Can you work these out from the model? Positions are in its coordinate system, mm. Face numbers are marked on the shaded views. A direction names the side the tool comes from. Round coordinates to 2 decimals unless told otherwise and drop trailing zeros. Loops run counter-clockwise (first coordinate to the right, second up) from the corner with the lowest first, then second, coordinate; pieces in that order, holes last.
Autodesk Fusion 360 part; units mm, degrees
sketch "Sketch1" plane through (0, 0, 0) normal (0, 0, 1) x (1, 0, 0)
  circle A0 centre (0, -11.5) radius 2 construction
  circle A1 centre (0, 0) radius 12 construction
  circle A2 centre (0, -11.5) radius 1.5
  circle A3 centre (0, 0) radius 8.5
  line L0 (0, 0) -> (8.6603, -5)
  circle A4 centre (0, 0) radius 11.5
  line L1 (0, 0) -> (-8.6603, -5)
  circle A5 centre (0, 0) radius 10
  dimension "d4" = 1.5
  dimension "d5" = -1.5
  dimension "d6" = 2
  dimension "d7" = 0.5
  dimension "d8" = 20
  dimension "d9" = 3
extrude "Extrude1" add sketch "Sketch1" along normal blind 2 contours A2 A4 | A2 A4 | A2 A4 | A3 L0 L1 A5 | A3 L0 L1 | A3 L0 L1 picked at (-8.9789, -3.0313)
sketch "Sketch2" plane through (0, 0, 2) normal (0, 0, 1) x (-1, 0, 0)
  arc A0 (7.3612, 4.25) -> (-7.3612, 4.25) centre (0, 0) ccw
  line L0 (-7.3612, 4.25) -> (-8.6603, 5)
  arc A1 (8.6603, 5) -> (-8.6603, 5) centre (0, 0) ccw
  line L1 (8.6603, 5) -> (7.3612, 4.25)
  arc A2 (-1.4968, 11.4022) -> (1.4968, 11.4022) centre (0, 0) ccw
  arc A3 (1.4968, 11.4022) -> (-1.4968, 11.4022) centre (0, 11.5) ccw
  circle A4 centre (0, 0) radius 5
  dimension "d12" = 10
extrude "Extrude2" add sketch "Sketch2" along normal blind 4.5 contours A4
sketch "Sketch3" plane through (0, 0, 6.5) normal (0, 0, 1) x (-1, 0, 0)
  circle A0 centre (0, 0) radius 5
  line L0 (-2, 2) -> (2, 2)
  line L1 (2, 2) -> (2, -2)
  line L2 (2, -2) -> (-2, -2)
  line L3 (-2, -2) -> (-2, 2)
extrude "Extrude3" add sketch "Sketch3" along normal blind 3.5 contours L0 L1 L2 L3
sketch "Sketch4" plane through (0, 0, 0) normal (0, 0, -1) x (1, 0, 0)
  arc A0 (7.3612, 4.25) -> (-7.3612, 4.25) centre (0, 0) ccw
  line L0 (-7.3612, 4.25) -> (-8.6603, 5)
  arc A1 (8.6603, 5) -> (-8.6603, 5) centre (0, 0) ccw
  line L1 (8.6603, 5) -> (7.3612, 4.25)
  arc A2 (-1.4968, 11.4022) -> (1.4968, 11.4022) centre (0, 0) ccw
  arc A3 (1.4968, 11.4022) -> (-1.4968, 11.4022) centre (0, 11.5) ccw
  circle A4 centre (0, 0) radius 1.6
  line L2 (-1.5875, 2.7496) -> (-3.175, 0)
  line L3 (-3.175, 0) -> (-1.5875, -2.7496)
  line L4 (-1.5875, -2.7496) -> (1.5875, -2.7496)
  line L5 (1.5875, -2.7496) -> (3.175, 0)
  line L6 (3.175, 0) -> (1.5875, 2.7496)
  line L7 (1.5875, 2.7496) -> (-1.5875, 2.7496)
  dimension "d17" = 3.2
  dimension "d20" = 3.175
extrude "Extrude4" cut sketch "Sketch4" against normal blind 3 contours L2 L3 L4 L5 L6 L7
extrude "Extrude5" cut 1 faces at (0.5286, -0.5507, 0) along direction (0, 0, 1) blind 10
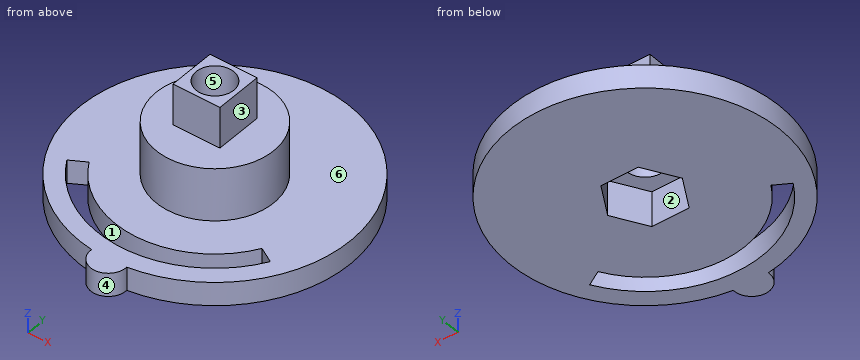
(1) If we section it at B-B, the plane x = 8: List the corners of the cut face in (y, z) for me.
Worked answers:
outline: (-8.26, 0) - (-6, 0) - (-6, 2) - (-8.26, 2) - close; (-4.62, 0) - (8.26, 0) - (8.26, 2) - (-4.62, 2) - close
(2) If we section it at A-A, the plane x = 0: List the corners of the cut face in (y, z) for me.
Worked answers:
outline: (-13, 0) - (-10, 0) - (-10, 2) - (-13, 2) - close; (-8.5, 0) - (-2.75, 0) - (-2.75, 3) - (-1.6, 3) - (-1.6, 10) - (-2, 10) - (-2, 6.5) - (-5, 6.5) - (-5, 2) - (-8.5, 2) - close; (1.6, 3) - (2.75, 3) - (2.75, 0) - (11.5, 0) - (11.5, 2) - (5, 2) - (5, 6.5) - (2, 6.5) - (2, 10) - (1.6, 10) - close
(3) For the marked faces 1, 2 and 3, which set-ups out of +Z, -Z, +X, -X, +Y, -Y let a thin tool reach every point of the face, with its end or its side?
Worked answers:
face 1: +Z, -Z
face 2: -Z
face 3: +Z, +X, +Y, -Y
(4) Will these pins go through, and if not, where does the flat tip stop? P1, Ø2, axis at x = 4, y = -2, coming from the +Z side; P2, Ø1.8, axis at y = 1, z = 7.5, coming from the -X side; P3, Ø2.5, axis at x = -0.5, z = 1.5, coming from the -Y side; P4, Ø6, axis at x = 6.5, z = 3.5, coming from the -Y side.
Worked answers:
P1: stops at z = 6.5
P2: stops at x = -2
P3: stops at y = -13
P4: stops at y = -10.82
(5) If we mould it in two halves opening along X, with no side actions, what happens to the marked faces 4, 5 and 6? For each: released by +X, released by -X, zero draft, split by the parting line, or undercut.
Worked answers:
face 4: split by the parting line
face 5: undercut
face 6: zero draft
(6) If I drill on line 1 (X direction, y = 0, z = 6); line 2 (Y direction, x = 0, z = 7.5); line 3 (Y direction, x = -2.75, z = 0.5), over which ranges is the centre line in solid material (lowest first)?
Worked answers:
line 1: x = -5 to -1.6, 1.6 to 5
line 2: y = -2 to -1.6, 1.6 to 2
line 3: y = -11.17 to -9.61, -8.04 to -0.74, 0.74 to 11.17
(7) If we section it at C-C, the plane y = -1: List the corners of the cut face in (x, z) for me.
Worked answers:
outline: (-11.46, 0) - (-2.6, 0) - (-2.6, 3) - (-1.25, 3) - (-1.25, 10) - (-2, 10) - (-2, 6.5) - (-4.9, 6.5) - (-4.9, 2) - (-11.46, 2) - close; (1.25, 3) - (2.6, 3) - (2.6, 0) - (11.46, 0) - (11.46, 2) - (4.9, 2) - (4.9, 6.5) - (2, 6.5) - (2, 10) - (1.25, 10) - close
(8) If we section it at D-D, the plane z = 4.75: List the corners of the cut face in (x, y) for me, then the cut area to 3 significant figures.
Worked answers:
outline: circle Ø10 at (0, 0); hole circle Ø3.2 at (0, 0)
area: 70.5 mm2
